```python
from build123d import *

# Parameters (mm, degrees)
F1_DEPTH = 20.32
F2_R     = 9.525
F3_DEPTH = 19.559


with BuildPart() as f1:
    # F0 (on Top) → F1 (new body)
    with BuildSketch(Plane.XY):
        with BuildLine():
            ThreePointArc((14.478, 7.747), (13.882841, 9.183841), (12.446, 9.779))
            Line((12.446, 9.779), (-12.446, 9.779))
            ThreePointArc((-12.446, 9.779), (-13.882841, 9.183841), (-14.478, 7.747))
            Line((-14.478, 7.747), (-14.478, -7.747))
            ThreePointArc((-14.478, -7.747), (-13.882841, -9.183841), (-12.446, -9.779))
            Line((-12.446, -9.779), (12.446, -9.779))
            ThreePointArc((12.446, -9.779), (13.882841, -9.183841), (14.478, -7.747))
            Line((14.478, -7.747), (14.478, 7.747))
        make_face()
        with BuildLine():
            Line((-12.446, 8.509), (12.446, 8.509))
            ThreePointArc((12.446, 8.509), (12.984815, 8.285815), (13.208, 7.747))
            Line((13.208, 7.747), (13.208, -7.747))
            ThreePointArc((13.208, -7.747), (12.984815, -8.285815), (12.446, -8.509))
            Line((12.446, -8.509), (-12.446, -8.509))
            ThreePointArc((-12.446, -8.509), (-12.984815, -8.285815), (-13.208, -7.747))
            Line((-13.208, -7.747), (-13.208, 7.747))
            ThreePointArc((-13.208, 7.747), (-12.984815, 8.285815), (-12.446, 8.509))
        make_face(mode=Mode.SUBTRACT)
    extrude(amount=F1_DEPTH)

    # F2 (on face) → F3 (cut, through all)
    with BuildSketch(Plane.XZ.offset(9.779)):
        with Locations((0, 20.32)):
            Circle(F2_R)
    extrude(amount=-F3_DEPTH, mode=Mode.SUBTRACT)


solid = f1.part
```
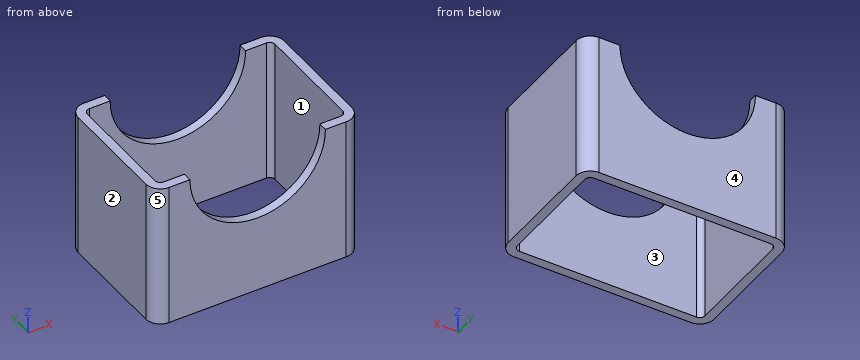
Can you work these out from the model? Positions are in its coordinate system, mm. Face numbers are marked on the shaded views. A direction names the side the tool comes from. Round coordinates to 2 decimals unless told otherwise and drop trailing zeros. Loops run counter-clockwise (first coordinate to the right, second up) from the corner with the lowest first, then second, coordinate; pieces in that order, holes last.
Item 1: Suppose I cut it at C-C, the plane x = 0. Write out the boundary of the cut face in (y, z) (3 decimals), then the cut area to 3 significant figures.
Item 2: Will this pin go through, and if not, where does the flat tip stop? pin 1 Ø6 at (x, z) = (-5, 13.5) entering from -Y.
Item 3: Please list where these lines run through material, in increasing order: L1, parallel to X at y = 0.5, z = 13.75; L2, parallel to Y at x = 8.5, z = 4.5; L3, parallel to Y at x = 13, z = 14.
Item 4: Suppose I cut it at A-A, the plane z = 1.5. Write out the boundary of the cut face in (x, y), then the cut area to 3 significant figures.
Item 5: Suppose I cut it at B-B, the plane y = -6.5. Write out the boundary of the cut face in (x, z).
Item 6: Which directions (+Z, -Z, +X, -X, +Y, -Y) give clear straight access to the entire face, cutting with the end or side of a thin tool? Please do the marked faces 1 and 2.
Item 7: If we mould it in two halves opening along Y, with no side actions, what happens to the marked faces 3, 4 and 5? For each: +Y half, -Y half, draft (parallel to the pull), parting line (faces both ways), or undercut.
Reported:
1. outline: (-9.779, 0) - (-8.509, 0) - (-8.509, 10.795) - (-9.779, 10.795) - close; (8.509, 0) - (9.779, 0) - (9.779, 10.795) - (8.509, 10.795) - close
1. area: 27.4 mm2
2. pin 1: stops at y = -9.78
3. L1: x = -14.48 to -13.21, 13.21 to 14.48
3. L2: y = -9.78 to -8.51, 8.51 to 9.78
3. L3: y = -9.7 to -8.27, 8.27 to 9.7
4. outline: (-14.48, -7.75) arc R2.03 ccw to (-12.45, -9.78) - (12.45, -9.78) arc R2.03 ccw to (14.48, -7.75) - (14.48, 7.75) arc R2.03 ccw to (12.45, 9.78) - (-12.45, 9.78) arc R2.03 ccw to (-14.48, 7.75) - close; hole (-13.21, -7.75) arc R0.76 ccw to (-12.45, -8.51) - (12.45, -8.51) arc R0.76 ccw to (13.21, -7.75) - (13.21, 7.75) arc R0.76 ccw to (12.45, 8.51) - (-12.45, 8.51) arc R0.76 ccw to (-13.21, 7.75) - close
4. area: 114 mm2
5. outline: (-14.48, 0) - (-13.21, 0) - (-13.21, 20.32) - (-14.48, 20.32) - close; (13.21, 0) - (14.48, 0) - (14.48, 20.32) - (13.21, 20.32) - close
6. face 1: +Z, -Z
6. face 2: +Z, -Z, -X, +Y, -Y
7. face 3: undercut
7. face 4: +Y half
7. face 5: -Y half
